Part model, mm, in its own coordinate system. Face numbers are marked on the shaded views. A direction names the side the tool comes from. Coordinates: 2 decimals unless noted, no trailing zeros. Loops run counter-clockwise (first coordinate to the right, second up) from the corner with the lowest first, then second, coordinate; pieces in that order, holes last. Notation, with made-up numbers: M -31.75,55 L 14.25,55 A35 cw 14.25,92 Z; hole C -17,-37 d7. An arc over 180 degrees is marked long. Answer as a JSON object with one key per item and string values. Group by question number.
1. Saw through at A-A on y = 12.5. Count the separate pieces of the cut face and the enclosed holes in it, then the cut area to 3 significant figures.
2. Drop flat-ended pins along their axis: pin 1 Ø6 at (y, z) = (3, 3.5) entering from +X; pin 2 Ø3 at (x, z) = (35, -0.5) entering from -Y; pin 3 Ø1 at (x, z) = (17, 4) entering from +Y. Give the stop position or say it passes through.
3. 3-axis set-ups, long thin cutter, end or side, ignore diameter. For the marked faces 5, 6, 7 and 8: which of +Z, -Z, +X, -X, +Y, -Y reach the whole face in a straight line?
4. Saw through at C-C on x = 22. Write the cut outline in (y, z), then the cut area to 3 significant figures.
5. Mould opens along X. For the marked faces 1, 2, 3 and 4 say: released by +X, released by -X, zero draft, split by the parting line, or undercut.
6. Saw through at B-B on y = 6. Write the cut outline in (x, z), then the cut area to 3 significant figures.
7. Drill centre lines: L1, parallel to Z at x = 0, y = 5; L2, parallel to X at y = -1.5, z = 2.5; L3, parallel to X at y = 2.5, z = -3.5. Where is each one in solid material? Low to high.
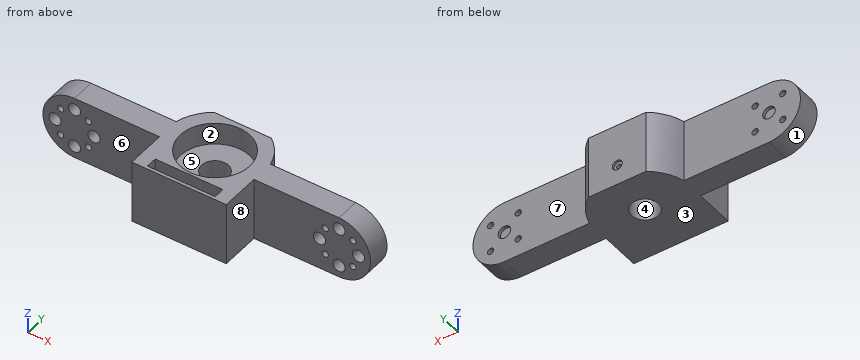
from build123d import *

# Parameters (mm, degrees)
BOSS_EXTRUDE1_DEPTH                                 = 25
SKETCH2_R                                           = 11.025
CUT_EXTRUDE1_DEPTH                                  = 7
CUT_EXTRUDE3_DEPTH                                  = 8.75
CUT_EXTRUDE5_DEPTH                                  = 8.75
SKETCH5_R                                           = 1
CUT_EXTRUDE6_DEPTH                                  = 7.5
SKETCH6_R                                           = 1.95
CUT_EXTRUDE7_DEPTH                                  = 6.5
SKETCH7_R                                           = 2
CUT_EXTRUDE8_DEPTH                                  = 1
CUT_EXTRUDE9_DEPTH                                  = 62.065538563
CUT_EXTRUDE10_REACH                                 = 61.144
SKETCH9_R                                           = 4.25
CBORE_FOR_00_BINDING_HEAD_MACHINE_SCREW_D           = 1.397
CBORE_FOR_00_BINDING_HEAD_MACHINE_SCREW_DEPTH       = 25
CBORE_FOR_00_BINDING_HEAD_MACHINE_SCREW_CBORE_D     = 3.175
CBORE_FOR_00_BINDING_HEAD_MACHINE_SCREW_CBORE_DEPTH = 0.7112
CBORE_FOR_00_BINDING_HEAD_MACHINE_SCREW_TIP         = 0.419701142
BOSS_EXTRUDE4_DEPTH                                 = 20
SKETCH20_W                                          = 21.5
SKETCH20_H                                          = 3.5
CUT_EXTRUDE13_DEPTH                                 = 16.5


with BuildPart() as part:
    # Sketch1 → Boss-Extrude1 (new body)
    with BuildSketch(Plane(origin=(0, 0, 0), x_dir=(1, 0, 0), z_dir=(0, 1, 0))):
        with BuildLine():
            Line((-42, -10), (42, -10))
            ThreePointArc((42, -10), (52, 0), (42, 10))
            Line((42, 10), (-42, 10))
            ThreePointArc((-42, 10), (-52, 0), (-42, -10))
        make_face()
    extrude(amount=BOSS_EXTRUDE1_DEPTH)

    # Sketch2 → Cut-Extrude1 (cut)
    with BuildSketch(Plane.XY.offset(10)):
        with Locations((0, 12.5)):
            Circle(SKETCH2_R)
    extrude(amount=-CUT_EXTRUDE1_DEPTH, mode=Mode.SUBTRACT)

    # Sketch3 → Cut-Extrude3 (cut)
    with BuildSketch(Plane.XZ):
        with BuildLine():
            Line((15, -10), (15, 10))
            Line((15, 10), (42, 10))
            ThreePointArc((42, 10), (52, 0), (42, -10))
            Line((42, -10), (15, -10))
        make_face()
        with BuildLine():
            Line((-15, -10), (-15, 10))
            Line((-15, 10), (-42, 10))
            ThreePointArc((-42, 10), (-52, 0), (-42, -10))
            Line((-42, -10), (-15, -10))
        make_face()
    extrude(amount=-CUT_EXTRUDE3_DEPTH, mode=Mode.SUBTRACT)

    # Sketch4 → Cut-Extrude5 (cut)
    with BuildSketch(Plane(origin=(0, 25, 0), x_dir=(1, 0, 0), z_dir=(0, 1, 0))):
        with BuildLine():
            Line((15, -10), (15, 10))
            Line((15, 10), (55, 10))
            ThreePointArc((55, 10), (65, 0), (55, -10))
            Line((55, -10), (15, -10))
        make_face()
        with BuildLine():
            Line((-15, -10), (-15, 10))
            Line((-15, 10), (-55, 10))
            ThreePointArc((-55, 10), (-65, 0), (-55, -10))
            Line((-55, -10), (-15, -10))
        make_face()
    extrude(amount=-CUT_EXTRUDE5_DEPTH, mode=Mode.SUBTRACT)

    # Sketch5 → Cut-Extrude6 (cut)
    with BuildSketch(Plane(origin=(0, 16.25, 0), x_dir=(1, 0, 0), z_dir=(0, 1, 0))):
        with Locations(Location((-46.384062043, 4.384062043, 0), (0, 0, 270))):
            Circle(SKETCH5_R)
        with Locations(Location((-37.615937957, 4.384062043, 0), (0, 0, 270))):
            Circle(SKETCH5_R)
        with Locations(Location((-37.615937957, -4.384062043, 0), (0, 0, 270))):
            Circle(SKETCH5_R)
        with Locations(Location((-46.384062043, -4.384062043, 0), (0, 0, 270))):
            Circle(SKETCH5_R)
        with Locations(Location((37.615937957, 4.384062043, 0), (0, 0, 270))):
            Circle(SKETCH5_R)
        with Locations(Location((46.384062043, 4.384062043, 0), (0, 0, 270))):
            Circle(SKETCH5_R)
        with Locations(Location((46.384062043, -4.384062043, 0), (0, 0, 270))):
            Circle(SKETCH5_R)
        with Locations(Location((37.615937957, -4.384062043, 0), (0, 0, 270))):
            Circle(SKETCH5_R)
    extrude(amount=-CUT_EXTRUDE6_DEPTH, mode=Mode.SUBTRACT)

    # Sketch6 → Cut-Extrude7 (cut)
    with BuildSketch(Plane.XZ.offset(-8.75)):
        with Locations(Location((-42, 6.2, 0), (0, 0, 270))):
            Circle(SKETCH6_R)
        with Locations(Location((-35.8, 0, 0), (0, 0, 270))):
            Circle(SKETCH6_R)
        with Locations(Location((-48.2, 0, 0), (0, 0, 270))):
            Circle(SKETCH6_R)
        with Locations(Location((-42, -6.2, 0), (0, 0, 270))):
            Circle(SKETCH6_R)
        with Locations(Location((42, 6.2, 0), (0, 0, 270))):
            Circle(SKETCH6_R)
        with Locations(Location((48.2, 0, 0), (0, 0, 270))):
            Circle(SKETCH6_R)
        with Locations(Location((35.8, 0, 0), (0, 0, 270))):
            Circle(SKETCH6_R)
        with Locations(Location((42, -6.2, 0), (0, 0, 270))):
            Circle(SKETCH6_R)
    extrude(amount=-CUT_EXTRUDE7_DEPTH, mode=Mode.SUBTRACT)

    # Sketch7 → Cut-Extrude8 (cut)
    with BuildSketch(Plane(origin=(0, 16.25, 0), x_dir=(1, 0, 0), z_dir=(0, 1, 0))):
        with Locations(Location((-42, 0, 0), (0, 0, 270))):
            Circle(SKETCH7_R)
        with Locations(Location((42, 0, 0), (0, 0, 270))):
            Circle(SKETCH7_R)
    extrude(amount=-CUT_EXTRUDE8_DEPTH, mode=Mode.SUBTRACT)

    # Sketch8 → Cut-Extrude9 (cut, through all)
    with BuildSketch(Plane.XY.offset(10)):
        with BuildLine():
            Line((-15, 16.25), (-15, 25))
            Line((-15, 25), (-9.100137362, 25))
            ThreePointArc((-9.100137362, 25), (-12.819702813, 21.143941218), (-15, 16.25))
        make_face()
        with BuildLine():
            Line((15, 0), (9.100137362, 0))
            ThreePointArc((9.100137362, 0), (12.819702813, 3.856058782), (15, 8.75))
            Line((15, 8.75), (15, 0))
        make_face()
        with BuildLine():
            Line((15, 25), (9.100137362, 25))
            ThreePointArc((9.100137362, 25), (12.819702813, 21.143941218), (15, 16.25))
            Line((15, 16.25), (15, 25))
        make_face()
        with BuildLine():
            Line((-15, 0), (-15, 8.75))
            ThreePointArc((-15, 8.75), (-12.819702813, 3.856058782), (-9.100137362, 0))
            Line((-9.100137362, 0), (-15, 0))
        make_face()
    extrude(amount=-CUT_EXTRUDE9_DEPTH, mode=Mode.SUBTRACT)

    # Sketch9 → Cut-Extrude10 (cut, up to next)
    with BuildSketch(Plane.XY.offset(3), mode=Mode.PRIVATE) as cut_extrude10_sk1:
        with Locations((0, 12.5)):
            Circle(SKETCH9_R)
    cut_extrude10_tool1 = extrude(cut_extrude10_sk1.sketch, amount=-CUT_EXTRUDE10_REACH, mode=Mode.PRIVATE) & part.part
    add(cut_extrude10_tool1.solids().sort_by_distance((0, 12.5, 3))[0], mode=Mode.SUBTRACT)

    # CBORE for #00 Binding Head Machine Screw2
    with Locations(Plane(origin=(0, 25, 0), x_dir=(1, 0, 0), z_dir=(0, 1, 0))):
        with Locations((0, 3.5)):
            CounterBoreHole(CBORE_FOR_00_BINDING_HEAD_MACHINE_SCREW_D / 2, CBORE_FOR_00_BINDING_HEAD_MACHINE_SCREW_CBORE_D / 2, CBORE_FOR_00_BINDING_HEAD_MACHINE_SCREW_CBORE_DEPTH, depth=CBORE_FOR_00_BINDING_HEAD_MACHINE_SCREW_DEPTH)
            with Locations((0, 0, -(CBORE_FOR_00_BINDING_HEAD_MACHINE_SCREW_DEPTH + CBORE_FOR_00_BINDING_HEAD_MACHINE_SCREW_TIP / 2))):  # 118° drill point
                Cone(0, CBORE_FOR_00_BINDING_HEAD_MACHINE_SCREW_D / 2, CBORE_FOR_00_BINDING_HEAD_MACHINE_SCREW_TIP, mode=Mode.SUBTRACT)

    # Sketch19 → Boss-Extrude4 (add, through all)
    with BuildSketch(Plane(origin=(0, 0, -10), x_dir=(-1, 0, 0), z_dir=(0, 0, -1))):
        with BuildLine():
            Line((-9.100137362, 0), (9.100137362, 0))
            ThreePointArc((9.100137362, 0), (12.819702813, 3.856058782), (15, 8.75))
            Line((15, 8.75), (15, -3.75))
            Line((15, -3.75), (-15, -3.75))
            Line((-15, -3.75), (-15, 8.75))
            ThreePointArc((-15, 8.75), (-12.819702813, 3.856058782), (-9.100137362, 0))
        make_face()
    extrude(amount=-BOSS_EXTRUDE4_DEPTH)

    # Sketch20 → Cut-Extrude13 (cut)
    with BuildSketch(Plane.XY.offset(10)):
        with Locations((0, -1)):
            Rectangle(SKETCH20_W, SKETCH20_H)
    extrude(amount=-CUT_EXTRUDE13_DEPTH, mode=Mode.SUBTRACT)


solid = part.part
Outcome:
{
 "1": {"separate pieces": "2", "enclosed holes": "16", "area": "1,610 mm²"},
 "2": {"pin 1": "stops at x = 15", "pin 2": "stops at y = 8.75", "pin 3": "stops at y = 16.25"},
 "3": {"face 5": "+Z", "face 6": "+Z, -Z, -X, -Y", "face 7": "+Z, -Z, +X, +Y", "face 8": "+Z, -Z, +X, -Y"},
 "4": {"outline": "M 8.75,-10 L 16.25,-10 L 16.25,10 L 8.75,10 Z", "area": "150 mm²"},
 "5": {"face 1": "released by -X", "face 2": "undercut", "face 3": "zero draft", "face 4": "undercut"},
 "6": {"outline": "M -15,-10 L 15,-10 L 15,10 L 8.91,10 L 8.91,3 L -8.91,3 L -8.91,10 L -15,10 Z; hole C 0,-3.5 d1.4", "area": "474 mm²"},
 "7": {"L1": "z = -10 to -4.2, -2.8 to 3", "L2": "x = -15 to -10.75, 10.75 to 15", "L3": "x = -15 to -0.7, 0.7 to 15"}
}
